The listing builds one solid part. Answer for the finished solid, in the listing's coordinates (mm). Face numbers are marked on the shaded views. A direction names the side the tool comes from. Round coordinates to 2 decimals unless told otherwise and drop trailing zeros. Write each loop counter-clockwise with the first axis right and the second up, starting at its lowest first coordinate (ties: lowest second). Pieces come first, ordered by that corner, then holes. Notation, with made-up numbers: (-3.75, -8.75) - (33.25, -8.75) arc R10 cw to (33.25, 4.25) - close; hole circle Ø11 at (-14, 7). An arc over 180 degrees is marked (long way). Return JSON: item names as keys, results as strings. Group by question number.
(1) Determine the mould class of the marked faces 1, 2 and 3 for opening direction X: +X half, -X half, draft (parallel to the pull), parting line (faces both ways), or undercut.
(2) Each of these flat-tipped pins is pushed along its axis until it touches: pin 1 (3 mm diameter, centred on x = -35, y = -18, fed in from -Z); pin 2 (20.5 mm diameter, centred on x = 0, z = 25.4, fed in from -Y); pin 3 (6 mm diameter, centred on x = 15.5, y = 17, fed in from +Z); pin 4 (10 mm diameter, centred on x = 19.5, y = -4.5, fed in from -Z). Where does it stop, or does it pass through?
(3) Section C-C, the plane z = 14 is taken. Write down the section's boundary in (x, y) (3 decimals), then the cut area to 3 significant figures.
(4) Section A-A, the plane x = -30.5 is taken. Write down the section's boundary in (y, z), then the cut area to 3 significant figures.
(5) Find the intervals of material crossed by line 1 along Y through (x, z) = (23.5, 2); line 2 along Z through (x, y) = (18, 19.5); line 3 along Z through (x, y) = (0, 15) (3 decimals), in increasing order. Write a range as [from, to].
(6) Which of the six approach directions +Z, -Z, +X, -X, +Y, -Y give full straight-line access (tool end or side, diameter ignored) to the marked faces 4, 5 and 6?
(7) Section B-B, the plane y = 0 is taken. Write down the section's boundary in (x, z).
(8) Section D-D, the plane z = 33 is taken. Write down the section's boundary in (x, y).
```python
from build123d import *

# Parameters (mm, degrees)
F1_DEPTH = 12.7
F2_R     = 6.35
F3_DEPTH = 12.7


with BuildPart() as f1:
    # F0 (on Top) → F1 (new body)
    with BuildSketch(Plane.XY):
        with BuildLine():
            Line((15.875, -25.4), (31.75, -25.4))
            ThreePointArc((31.75, -25.4), (57.15, 0), (31.75, 25.4))
            Line((31.75, 25.4), (0, 25.4))
            Line((0, 25.4), (-31.75, 25.4))
            ThreePointArc((-31.75, 25.4), (-57.15, 0), (-31.75, -25.4))
            Line((-31.75, -25.4), (-15.875, -25.4))
            Line((-15.875, -25.4), (-15.875, -12.7))
            Line((-15.875, -12.7), (-31.75, -12.7))
            ThreePointArc((-31.75, -12.7), (-44.45, 0), (-31.75, 12.7))
            Line((-31.75, 12.7), (0, 12.7))
            Line((0, 12.7), (31.75, 12.7))
            ThreePointArc((31.75, 12.7), (44.45, 0), (31.75, -12.7))
            Line((31.75, -12.7), (15.875, -12.7))
            Line((15.875, -12.7), (15.875, -25.4))
        make_face()
    extrude(amount=F1_DEPTH)

    # F2 (on face) → F3 (join)
    with BuildSketch(Plane.XZ.offset(-12.7)):
        with BuildLine():
            Line((15.875, 0), (15.875, 25.4))
            ThreePointArc((15.875, 25.4), (0, 41.275), (-15.875, 25.4))
            Line((-15.875, 25.4), (-15.875, -0.097406))
            Line((-15.875, -0.097406), (15.875, 0))
        make_face()
        with Locations((0, 25.4)):
            Circle(F2_R, mode=Mode.SUBTRACT)
    extrude(amount=-F3_DEPTH)


solid = f1.part
```
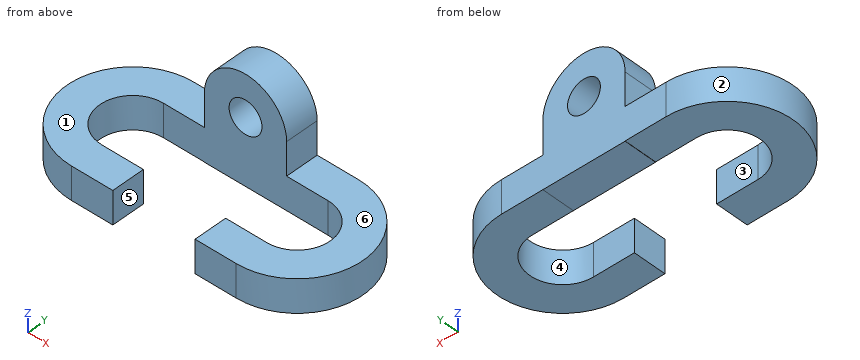
Working result:
{
 "1": {"face 1": "draft", "face 2": "-X half", "face 3": "undercut"},
 "2": {"pin 1": "stops at z = 0", "pin 2": "stops at y = 12.7", "pin 3": "stops at z = 35.19", "pin 4": "passes through"},
 "3": {"outline": "(-15.875, 12.7) - (15.875, 12.7) - (15.875, 25.4) - (-15.875, 25.4) - close", "area": "403 mm^2"},
 "4": {"outline": "(-25.4, 0) - (-12.7, 0) - (-12.7, 12.7) - (-25.4, 12.7) - close; (12.7, 0) - (25.4, 0) - (25.4, 12.7) - (12.7, 12.7) - close", "area": "323 mm^2"},
 "5": {"line 1": "y = [-25.4, -12.7], [12.7, 25.4]", "line 2": "z = [0, 12.7]", "line 3": "z = [-0.049, 19.05], [31.75, 41.275]"},
 "6": {"face 4": "+Z, -Z", "face 5": "+Z, -Z, -Y", "face 6": "+Z, +X, +Y, -Y"},
 "7": {"outline": "(-57.15, 0) - (-44.45, 0) - (-44.45, 12.7) - (-57.15, 12.7) - close; (44.45, 0) - (57.15, 0) - (57.15, 12.7) - (44.45, 12.7) - close"},
 "8": {"outline": "(-13.94, 12.7) - (13.94, 12.7) - (13.94, 25.4) - (-13.94, 25.4) - close"}
}
